Verification items for the finished model (mm, model axes). Give positions to 0.01 mm unless a question says otherwise; leave off trailing zeros. Loops run counter-clockwise (first coordinate to the right, second up) from the corner with the lowest first, then second, coordinate; pieces in that order, holes last. Notation, with made-up numbers: M 59,-27.5 L 117,-27.5 A15 cw 117,-15.5 Z; hole C -7,55.5 d1. An arc over 180 degrees is marked long. Put each result on its own line as item: value. Start each with the question number.
from build123d import *

# Parameters (mm, degrees)
SKETCH_1_W          = 10
SKETCH_1_H          = 10
SKETCH_1_W_2        = 8
SKETCH_1_H_2        = 8
EXTRUDE_1_DEPTH     = 100
SKETCH_2_R          = 1.6
CUT_EXTRUDE_1_DEPTH = 101.623058987
SKETCH_3_R          = 1.6
CUT_EXTRUDE_2_DEPTH = 100


with BuildPart() as part:
    # ｽｹｯﾁ1 → ﾎﾞｽ - 押し出し1 (new body)
    with BuildSketch(Plane.XY):
        Rectangle(SKETCH_1_W, SKETCH_1_H)
        Rectangle(SKETCH_1_W_2, SKETCH_1_H_2, mode=Mode.SUBTRACT)
    extrude(amount=EXTRUDE_1_DEPTH)

    # ｽｹｯﾁ2 → ｶｯﾄ - 押し出し1 (cut, through all)
    with BuildSketch(Plane(origin=(5, 0, 0), x_dir=(0, 0, -1), z_dir=(1, 0, 0))):
        with Locations(Location((-85, 0, 0), (0, 0, 90))):
            Circle(SKETCH_2_R)
        with Locations(Location((-15, 0, 0), (0, 0, 90))):
            Circle(SKETCH_2_R)
    extrude(amount=-CUT_EXTRUDE_1_DEPTH, mode=Mode.SUBTRACT)

    # ｽｹｯﾁ3 → ｶｯﾄ - 押し出し2 (cut)
    with BuildSketch(Plane(origin=(0, 5, 0), x_dir=(1, 0, 0), z_dir=(0, 1, 0))):
        with Locations(Location((0, -95, 0), (0, 0, 270))):
            Circle(SKETCH_3_R)
        with Locations(Location((0, -5, 0), (0, 0, 270))):
            Circle(SKETCH_3_R)
    extrude(amount=-CUT_EXTRUDE_2_DEPTH, mode=Mode.SUBTRACT)


solid = part.part
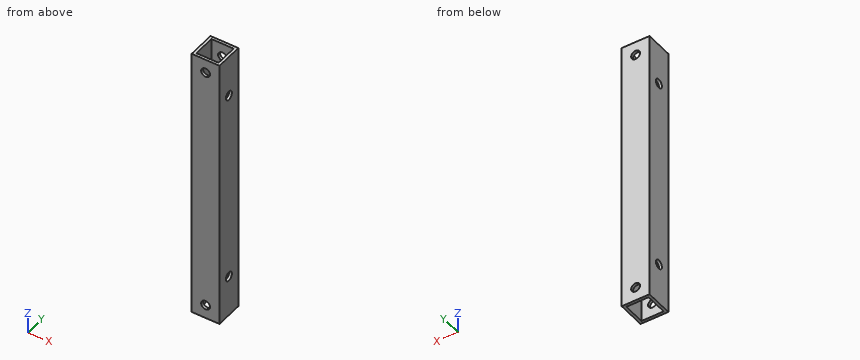
Q1. Cross-section at D-D, the plane z = 5. Record the boundary of the cut face in (x, y), then the cut area to 3 significant figures.
Q2. Cross-section at C-C, the plane y = 0. Record the boundary of the cut face in (x, z), then the cut area to 3 significant figures.
Q3. Go/stop test with flat-tipped pins: pin 1 (3 mm diameter, centred on x = 1, y = -3, fed in from -Z); pin 2 (3 mm diameter, centred on y = 0, z = 15, fed in from -X). Record where each tip stops, or that it passes through.
Q4. Scan lines: L1, parallel to Z at x = 4.4, y = 0; L2, parallel to Y at x = -3.75, z = 82.5. Record each from-to range of solid material in increasing order.
Q5. Cross-section at A-A, the plane x = 0. Record the boundary of the cut face in (y, z).
Q6. Cross-section at B-B, the plane z = 68.5. Record the boundary of the cut face in (x, y).
Ans:
1. outline: M -5,-5 L -1.6,-5 L -1.6,-4 L -4,-4 L -4,4 L -1.6,4 L -1.6,5 L -5,5 Z; M 1.6,-5 L 5,-5 L 5,5 L 1.6,5 L 1.6,4 L 4,4 L 4,-4 L 1.6,-4 Z
1. area: 29.6 mm^2
2. outline: M -5,0 L -4,0 L -4,13.4 L -5,13.4 Z; M -5,16.6 L -4,16.6 L -4,83.4 L -5,83.4 Z; M -5,86.6 L -4,86.6 L -4,100 L -5,100 Z; M 4,0 L 5,0 L 5,13.4 L 4,13.4 Z; M 4,16.6 L 5,16.6 L 5,83.4 L 4,83.4 Z; M 4,86.6 L 5,86.6 L 5,100 L 4,100 Z
2. area: 187 mm^2
3. pin 1: stops at z = 0
3. pin 2: passes through
4. L1: z = 0 to 13.4, 16.6 to 83.4, 86.6 to 100
4. L2: y = -5 to -4, 4 to 5
5. outline: M -5,0 L -4,0 L -4,3.4 L -5,3.4 Z; M -5,6.6 L -4,6.6 L -4,93.4 L -5,93.4 Z; M -5,96.6 L -4,96.6 L -4,100 L -5,100 Z; M 4,0 L 5,0 L 5,3.4 L 4,3.4 Z; M 4,6.6 L 5,6.6 L 5,93.4 L 4,93.4 Z; M 4,96.6 L 5,96.6 L 5,100 L 4,100 Z
6. outline: M -5,-5 L 5,-5 L 5,5 L -5,5 Z; hole M -4,-4 L 4,-4 L 4,4 L -4,4 Z
